Check sheet for the modelled part. Datum: model origin and axes. Units: mm. Give positions to 0.01 mm unless a question says otherwise; leave off trailing zeros. Order: outer loops, then holes, each group sorted by start corner. A loop starts at its lowest first (then second) coordinate and runs counter-clockwise, first axis right, second up.
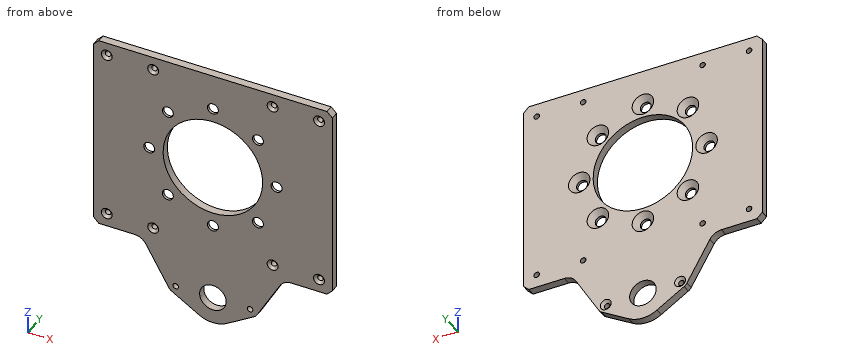
```python
from build123d import *

# Parameters (mm, degrees)
SKETCH_1_W          = 180
SKETCH_1_H          = 150
SKETCH_1_R          = 4.1
SKETCH_1_R_2        = 2.1
EXTRUDE_1_DEPTH     = 3
CHAMFER_1_SIZE      = 4
CHAMFER_2_SIZE      = 4
CHAMFER_3_SIZE      = 2
SKETCH_3_R          = 37.5
CUT_EXTRUDE_1_DEPTH = 118.307288776
SKETCH_4_R          = 2.1
SKETCH_4_R_2        = 10
EXTRUDE_2_DEPTH     = 6
CHAMFER_4_SIZE      = 2
FILLET_1_R          = 10


with BuildPart() as part:
    # 草图1 → 凸台-拉伸1 (new, symmetric)
    with BuildSketch(Plane(origin=(0, 0, 0), x_dir=(1, 0, 0), z_dir=(0, 1, 0))):
        Rectangle(SKETCH_1_W, SKETCH_1_H)
        with Locations(Location((0, 48, 0), (0, 0, 270))):
            Circle(SKETCH_1_R, mode=Mode.SUBTRACT)
        with Locations(Location((33.941125497, 33.941125497, 0), (0, 0, 270))):
            Circle(SKETCH_1_R, mode=Mode.SUBTRACT)
        with Locations(Location((48, 0, 0), (0, 0, 270))):
            Circle(SKETCH_1_R, mode=Mode.SUBTRACT)
        with Locations(Location((33.941125497, -33.941125497, 0), (0, 0, 270))):
            Circle(SKETCH_1_R, mode=Mode.SUBTRACT)
        with Locations(Location((0, -48, 0), (0, 0, 270))):
            Circle(SKETCH_1_R, mode=Mode.SUBTRACT)
        with Locations(Location((-33.941125497, -33.941125497, 0), (0, 0, 270))):
            Circle(SKETCH_1_R, mode=Mode.SUBTRACT)
        with Locations(Location((-48, 0, 0), (0, 0, 270))):
            Circle(SKETCH_1_R, mode=Mode.SUBTRACT)
        with Locations(Location((-33.941125497, 33.941125497, 0), (0, 0, 270))):
            Circle(SKETCH_1_R, mode=Mode.SUBTRACT)
        with Locations(Location((-80, 65, 0), (0, 0, 270))):
            Circle(SKETCH_1_R_2, mode=Mode.SUBTRACT)
        with Locations(Location((-45, 65, 0), (0, 0, 270))):
            Circle(SKETCH_1_R_2, mode=Mode.SUBTRACT)
        with Locations(Location((45, 65, 0), (0, 0, 90))):
            Circle(SKETCH_1_R_2, mode=Mode.SUBTRACT)
        with Locations(Location((80, 65, 0), (0, 0, 90))):
            Circle(SKETCH_1_R_2, mode=Mode.SUBTRACT)
        with Locations(Location((80, -65, 0), (0, 0, 270))):
            Circle(SKETCH_1_R_2, mode=Mode.SUBTRACT)
        with Locations(Location((45, -65, 0), (0, 0, 270))):
            Circle(SKETCH_1_R_2, mode=Mode.SUBTRACT)
        with Locations(Location((-45, -65, 0), (0, 0, 90))):
            Circle(SKETCH_1_R_2, mode=Mode.SUBTRACT)
        with Locations(Location((-80, -65, 0), (0, 0, 90))):
            Circle(SKETCH_1_R_2, mode=Mode.SUBTRACT)
    extrude(amount=EXTRUDE_1_DEPTH, both=True)

    # 倒角1
    chamfer_1_edges = [part.edges().sort_by_distance(p)[0] for p in [
        (0, 3, -52.1),
        (33.941125497, 3, -38.041125497),
        (48, 3, -4.1),
        (33.941125497, 3, 29.841125497),
        (0, 3, 43.9),
        (-33.941125497, 3, 29.841125497),
        (-48, 3, -4.1),
        (-33.941125497, 3, -38.041125497),
    ]]
    chamfer(chamfer_1_edges, length=CHAMFER_1_SIZE)

    # 倒角2
    chamfer_2_edges = [part.edges().sort_by_distance(p)[0] for p in [
        (90, 0, 75),
        (-90, 0, 75),
        (-90, 0, -75),
        (90, 0, -75),
    ]]
    chamfer(chamfer_2_edges, length=CHAMFER_2_SIZE)

    # 倒角3
    chamfer_3_edges = [part.edges().sort_by_distance(p)[0] for p in [
        (-80, -3, -67.1),
        (-45, -3, -67.1),
        (45, -3, -62.9),
        (80, -3, -62.9),
        (80, -3, 62.9),
        (45, -3, 62.9),
        (-45, -3, 67.1),
        (-80, -3, 67.1),
    ]]
    chamfer(chamfer_3_edges, length=CHAMFER_3_SIZE)

    # 草图3 → 切除-拉伸1 (cut, through all)
    with BuildSketch(Plane.XZ.offset(3)):
        with Locations(Location((0, 0, 0), (0, 0, 270))):
            Circle(SKETCH_3_R)
    extrude(amount=-CUT_EXTRUDE_1_DEPTH, mode=Mode.SUBTRACT)

    # 草图4 → 凸台-拉伸2 (add)
    with BuildSketch(Plane.XZ.offset(3)):
        with BuildLine():
            Line((-31.107142857, -112.132802672), (-10.616071429, -124.537075795))
            ThreePointArc((-10.616071429, -124.537075795), (0, -127.5), (10.616071429, -124.537075795))
            Line((10.616071429, -124.537075795), (31.107142857, -112.132802672))
            ThreePointArc((31.107142857, -112.132802672), (32.286419244, -111.198405658), (33.196152423, -110))
            Line((33.196152423, -110), (53.403411844, -75))
            Line((53.403411844, -75), (-53.403411844, -75))
            Line((-53.403411844, -75), (-33.196152423, -110))
            ThreePointArc((-33.196152423, -110), (-32.286419244, -111.198405658), (-31.107142857, -112.132802672))
        make_face()
        with Locations(Location((-28, -107, 0), (0, 0, 270))):
            Circle(SKETCH_4_R, mode=Mode.SUBTRACT)
        with Locations(Location((28, -107, 0), (0, 0, 270))):
            Circle(SKETCH_4_R, mode=Mode.SUBTRACT)
        with Locations(Location((0, -107, 0), (0, 0, 270))):
            Circle(SKETCH_4_R_2, mode=Mode.SUBTRACT)
    extrude(amount=-EXTRUDE_2_DEPTH)

    # 倒角4
    chamfer_4_edges = [part.edges().sort_by_distance(p)[0] for p in [
        (28, 3, -104.9),
        (-28, 3, -104.9),
    ]]
    chamfer(chamfer_4_edges, length=CHAMFER_4_SIZE)

    # 圆角1
    fillet_1_edges = [part.edges().sort_by_distance(p)[0] for p in [
        (-53.403411844, 0, -75),
        (53.403411844, 0, -75),
    ]]
    fillet(fillet_1_edges, radius=FILLET_1_R)


solid = part.part
```
(1) Cross-section at A-A on z = 48. Enter the section's corners in (x, y).
Response values:
outline: (-90, -3) - (-4.1, -3) - (-4.1, -1) - (-8.1, 3) - (-90, 3) - close; (4.1, -3) - (90, -3) - (90, 3) - (8.1, 3) - (4.1, -1) - close
(2) Cross-section at D-D on z = -21. Enter the section's corners in (x, y).
Response values:
outline: (-90, -3) - (-31.07, -3) - (-31.07, 3) - (-90, 3) - close; (31.07, -3) - (90, -3) - (90, 3) - (31.07, 3) - close
(3) Cross-section at C-C on z = 0. Enter the section's corners in (x, y), then the cut area to 3 significant figures.
Response values:
outline: (-90, -3) - (-52.1, -3) - (-52.1, -1) - (-56.1, 3) - (-90, 3) - close; (-43.9, -3) - (-37.5, -3) - (-37.5, 3) - (-39.9, 3) - (-43.9, -1) - close; (37.5, -3) - (43.9, -3) - (43.9, -1) - (39.9, 3) - (37.5, 3) - close; (52.1, -3) - (90, -3) - (90, 3) - (56.1, 3) - (52.1, -1) - close
area: 500 mm2
(4) Material ranges on L1, parallel to X at y = 0.85, z = -65; L2, parallel to X at y = -1.5, z = 0; L3, parallel to X at y = -2.3, z = -48, recorded low to high.
Response values:
L1: x = -90 to -82.1, -77.9 to -47.1, -42.9 to 42.9, 47.1 to 77.9, 82.1 to 90
L2: x = -90 to -52.1, -43.9 to -37.5, 37.5 to 43.9, 52.1 to 90
L3: x = -90 to -4.1, 4.1 to 90
(5) Gauge pin test, flat ends, axial feed: pin 1 Ø7.5 at (x, z) = (33.94, 33.94) entering from -Y; pin 2 Ø1.5 at (x, y) = (30, 0.5) entering from -Z; pin 3 Ø10.5 at (x, z) = (-33.94, -33.94) entering from +Y; pin 4 Ø5 at (x, z) = (80, -65) entering from -Y. Record the tip position at first contact, or that the pin passes through.
Response values:
pin 1: passes through
pin 2: stops at z = -113.26
pin 3: stops at y = 0.15
pin 4: stops at y = -1.4
(6) Cross-section at B-B on x = 0. Enter the section's corners in (y, z), then the cut area to 3 significant figures.
Response values:
outline: (-3, -127.5) - (3, -127.5) - (3, -117) - (-3, -117) - close; (-3, -97) - (3, -97) - (3, -56.1) - (-1, -52.1) - (-3, -52.1) - close; (-3, -43.9) - (-1, -43.9) - (3, -39.9) - (3, -37.5) - (-3, -37.5) - close; (-3, 37.5) - (3, 37.5) - (3, 39.9) - (-1, 43.9) - (-3, 43.9) - close; (-3, 52.1) - (-1, 52.1) - (3, 56.1) - (3, 75) - (-3, 75) - close
area: 515 mm2
